Work out the finished part from the listing and answer in its coordinate system (mm). A direction names the side the tool comes from. Give positions to 0.01 mm unless a question says otherwise; leave off trailing zeros. Loops run counter-clockwise (first coordinate to the right, second up) from the corner with the lowest first, then second, coordinate; pieces in that order, holes last. Notation, with made-up numbers: (50, -21) - (57, -21) arc R9 cw to (57, -5) - close; hole circle Ø3 at (78, -17). An arc over 180 degrees is marked (long way). One line per item, written item: value.
from build123d import *

# Parameters (mm, degrees)
F0_W     = 14
F0_H     = 8
F1_DEPTH = 5
F4_START = -1
F2_R     = 2
F4_DEPTH = 6
F5_DEPTH = 25
F7_DEPTH = 5


with BuildPart() as f1:
    # F0 (on Top) → F1 (new body)
    with BuildSketch(Plane.XY):
        with Locations((-5.3940967023, -6.1688271388)):
            Rectangle(F0_W, F0_H)
    extrude(amount=F1_DEPTH)

    # F2 (on face) → F4 (cut)
    with BuildSketch(Plane.XZ.offset(10.1688271388).offset(F4_START)):
        with Locations((-5.3940967023, 5)):
            Circle(F2_R)
    extrude(amount=-F4_DEPTH, mode=Mode.SUBTRACT)

    # F3 (on face) → F5 (cut)
    with BuildSketch(Plane.XZ.offset(10.1688271388)):
        with BuildLine():
            ThreePointArc((-6.8940967023, 5), (-5.3940967023, 6.5), (-3.8940967023, 5))
            Line((-3.8940967023, 5), (-3.3940967023, 5))
            ThreePointArc((-3.3940967023, 5), (-5.3940967023, 7), (-7.3940967023, 5))
            Line((-7.3940967023, 5), (-6.8940967023, 5))
        make_face()
        with BuildLine():
            ThreePointArc((-6.8940967023, 5), (-5.3940967023, 3.5), (-3.8940967023, 5))
            Line((-3.8940967023, 5), (-6.8940967023, 5))
        make_face()
        with BuildLine():
            Line((-6.8940967023, 5), (-3.8940967023, 5))
            ThreePointArc((-3.8940967023, 5), (-5.3940967023, 6.5), (-6.8940967023, 5))
        make_face()
    extrude(amount=-F5_DEPTH, mode=Mode.SUBTRACT)

    # F6 (on face) → F7 (cut)
    with BuildSketch(Plane.XY.offset(5)):
        with BuildLine():
            ThreePointArc((-11.3940967023, -6.1688271388), (-9.8940967023, -7.6688271388), (-8.3940967023, -6.1688271388))
            Line((-8.3940967023, -6.1688271388), (-11.3940967023, -6.1688271388))
        make_face()
        with BuildLine():
            Line((-11.3940967023, -6.1688271388), (-8.3940967023, -6.1688271388))
            ThreePointArc((-8.3940967023, -6.1688271388), (-9.8940967023, -4.6688271388), (-11.3940967023, -6.1688271388))
        make_face()
        with BuildLine():
            ThreePointArc((0.6059032977, -6.1688271388), (-0.8940967023, -4.6688271388), (-2.3940967023, -6.1688271388))
            Line((-2.3940967023, -6.1688271388), (0.6059032977, -6.1688271388))
        make_face()
        with BuildLine():
            Line((0.6059032977, -6.1688271388), (-2.3940967023, -6.1688271388))
            ThreePointArc((-2.3940967023, -6.1688271388), (-0.8940967023, -7.6688271388), (0.6059032977, -6.1688271388))
        make_face()
    extrude(amount=-F7_DEPTH, mode=Mode.SUBTRACT)


solid = f1.part
1. Section A-A (x = -1.5) is taken. Write down the section's boundary in (y, z), and give its area (3 significant figures).
Output:
outline: (-10.17, 0) - (-7.54, 0) - (-7.54, 5) - (-10.17, 5) - close; (-4.8, 0) - (-2.17, 0) - (-2.17, 5) - (-4.8, 5) - close
area: 26.3 mm²
2. Section D-D (y = -3) is taken. Write down the section's boundary in (x, z).
Output:
outline: (-12.39, 0) - (1.61, 0) - (1.61, 5) - (-3.89, 5) arc R1.5 cw to (-6.89, 5) - (-12.39, 5) - close
3. For faces 1 (the flat face through (-5, -10.169, 2)), 2 (the flat face through (-5.6, -3.169, 3.3)), determine the directions among +Z, -Z, +X, -X, +Y, -Y from which every point of the face is accessible in a straight line to the end or side of a thin tool.
Output:
face 1: +Z, -Z, +X, -X, -Y
face 2: +Z
4. Section B-B (z = 4.65) is taken. Write down the section's boundary in (x, y).
Output:
outline: (-12.39, -10.17) - (-6.85, -10.17) - (-6.85, -9.17) - (-7.36, -9.17) - (-7.36, -3.17) - (-6.85, -3.17) - (-6.85, -2.17) - (-12.39, -2.17) - close; (-3.94, -10.17) - (1.61, -10.17) - (1.61, -2.17) - (-3.94, -2.17) - (-3.94, -3.17) - (-3.42, -3.17) - (-3.42, -9.17) - (-3.94, -9.17) - close; hole circle Ø3 at (-9.89, -6.17); hole circle Ø3 at (-0.89, -6.17)
5. A flat-ended cylindrical pin translates along its axis: pin 1 Ø0.6 at (x, z) = (-6, 4.5) entering from +Y. Find the tip coordinate at first contact, or state that the pin passes through.
Output:
pin 1: passes through
6. Find the intervals of material crossed by line 1 along X through (y, z) = (-4.5, 3.2); line 2 along Y through (x, z) = (-5.5, 3.3); line 3 along X through (y, z) = (-2.5, 4.75), in increasing order.
Output:
line 1: x = -12.39 to -6.27, -4.52 to 1.61
line 2: y = -10.17 to -9.17, -3.17 to -2.17
line 3: x = -12.39 to -6.87, -3.92 to 1.61
7. The mould has two halves that part along X. Classify faces 3 (the flat face through (-5, -6, 0)), 4 (the cylindrical face through (-8.463, -5.718, 2.535)), 5 (the flat face through (1.606, -6, 2)): released by +X, released by -X, zero draft, split by the parting line, or undercut.
Output:
face 3: zero draft
face 4: undercut
face 5: released by +X
8. Section C-C (y = -6.5) is taken. Write down the section's boundary in (x, z).
Output:
outline: (-12.39, 0) - (-11.36, 0) - (-11.36, 5) - (-12.39, 5) - close; (-8.43, 0) - (-2.36, 0) - (-2.36, 5) - (-3.39, 5) arc R2 cw to (-7.39, 5) - (-8.43, 5) - close; (0.57, 0) - (1.61, 0) - (1.61, 5) - (0.57, 5) - close
